Design review of the part built by this model. Coordinates are the model's own, in mm. A direction names the side the tool comes from. Coordinates: 2 decimals unless noted, no trailing zeros. Write each loop counter-clockwise with the first axis right and the second up, starting at its lowest first coordinate (ties: lowest second). Pieces come first, ordered by that corner, then holes. Notation, with made-up numbers: M 81,24 L 111,24 A20 ccw 111,38 Z; hole C 45.25,-17 d9. An arc over 180 degrees is marked long. One line per question, with ' | ' between items.
from build123d import *

# Parameters (mm, degrees)
EKSTR_ZYON_NCE1_DEPTH = 66


with BuildPart() as part:
    # Çizim1 → Ekstrüzyon-İnce1 (new body)
    with BuildSketch(Plane.XY):
        Polygon((-58.502445294, 23.386048527), (-27.071596074, -46.959185442), (63.105007045, -46.959185442), (101.271038241, 23.386048527), (105.665865377, 21.001621038), (66.080746967, -51.959185442), (-30.313952532, -51.959185442), (-63.067488848, 21.346348216), align=None)
    extrude(amount=EKSTR_ZYON_NCE1_DEPTH)


solid = part.part
1. Tool access review of faces 1 (the face through (-46.46, -15.82, 32.54)), 2 (the face through (-43.01, -11.29, 32.54)): name each direction out of +Z, -Z, +X, -X, +Y, -Y from which nothing blocks a thin tool from reaching the whole face with its end or side.
Answer sheet:
face 1: +Z, -Z, -X, -Y | face 2: +Z, -Z, +Y
2. Take a section at B-B (z = 31). Write out the cut boundary in (x, y) (3 decimals), then the cut area to 3 significant figures.
Answer sheet:
outline: M -63.067,21.346 L -30.314,-51.959 L 66.081,-51.959 L 105.666,21.002 L 101.271,23.386 L 63.105,-46.959 L -27.072,-46.959 L -58.502,23.386 Z | area: 1,270 mm^2
3. Take a section at A-A (y = -21). Write out the cut boundary in (x, z), then the cut area to 3 significant figures.
Answer sheet:
outline: M -44.15,0 L -38.67,0 L -38.67,66 L -44.15,66 Z; M 77.19,0 L 82.88,0 L 82.88,66 L 77.19,66 Z | area: 737 mm^2
4. To check wall thickness, follow line 1 along Y through (x, z) = (38.5, 16.5); line 2 along X through (y, z) = (-37.5, 63); line 3 along X through (y, z) = (-11.5, 31.5). State the ranges of each line that lie inside material, in increasing order. Write a range as [from, to].
Answer sheet:
line 1: [-51.96, -46.96] | line 2: [-36.77, -31.3], [68.24, 73.93] | line 3: [-48.39, -42.92], [82.34, 88.03]
5. Draft analysis for pull direction X (two halves, no side actions). For faces 3 (the face through (19, -51.959, 33)), 4 (the face through (86.15, -14.97, 32.54)), 5 (the face through (17, -46.959, 33)), state which applies: pulls with the +X half, pulls with the -X half, needs draft (parallel to the pull), parting line crosses it, or undercut.
Answer sheet:
face 3: needs draft | face 4: pulls with the +X half | face 5: undercut
6. Take a section at C-C (x = -19). Write out the cut boundary in (y, z).
Answer sheet:
outline: M -51.96,0 L -46.96,0 L -46.96,66 L -51.96,66 Z
7. Insertion check: pin 1 Ø1.5 at (y, z) = (-38.5, 57) entering from -X; pin 2 Ø20 at (x, z) = (5.5, 23.5) entering from +Y; pin 3 Ø2 at (y, z) = (7.5, 39) entering from -X. Each pin has a flat end and moves straight along its axis. Give the tip position at first contact, or say it passes through.
Answer sheet:
pin 1: x = -36.66 | pin 2: y = -46.96 | pin 3: x = -57.33
